```python
from build123d import *

# Parameters (mm, degrees)
F0_R     = 1
F1_DEPTH = 8
F0_W     = 23
F0_H     = 6
F2_DEPTH = 20
F4_START = -1.8
F3_W     = 10
F3_H     = 10
F3_R     = 3
F4_DEPTH = 6


with BuildPart() as f1:
    # F0 (on Top) → F1 (new body)
    with BuildSketch(Plane.XY):
        Polygon((-11.5, 1.7857142857), (-11.5, 7.7857142857), (-16.5, 7.7857142857), (-16.5, -10.2142857143), (-11.5, -10.2142857143), align=None)
        with Locations((-14, -4.7142857143)):
            Circle(F0_R, mode=Mode.SUBTRACT)
    extrude(amount=F1_DEPTH)



with BuildPart() as f1b:
    # F0 (on Top) → F1, piece 2 (new body)
    with BuildSketch(Plane.XY):
        Polygon((16.5, 7.7857142857), (11.5, 7.7857142857), (11.5, 1.7857142857), (11.5, -10.2142857143), (16.5, -10.2142857143), align=None)
        with Locations((14, -4.7142857143)):
            Circle(F0_R, mode=Mode.SUBTRACT)
    extrude(amount=F1_DEPTH)


with BuildPart() as f1_1:
    add(f1.part)

    add(f1b.part)  # F2 merges F1b
    # F0 (on Top) → F2 (join)
    with BuildSketch(Plane.XY):
        with Locations((0, 4.7857142857)):
            Rectangle(F0_W, F0_H)
    extrude(amount=F2_DEPTH)

    # F3 (on Front) → F4 (join)
    with BuildSketch(Plane.XZ.offset(F4_START)):
        with Locations((0, 25)):
            Rectangle(F3_W, F3_H)
        with Locations((0, 25)):
            Circle(F3_R, mode=Mode.SUBTRACT)
    extrude(amount=-F4_DEPTH)


solid = f1_1.part
```
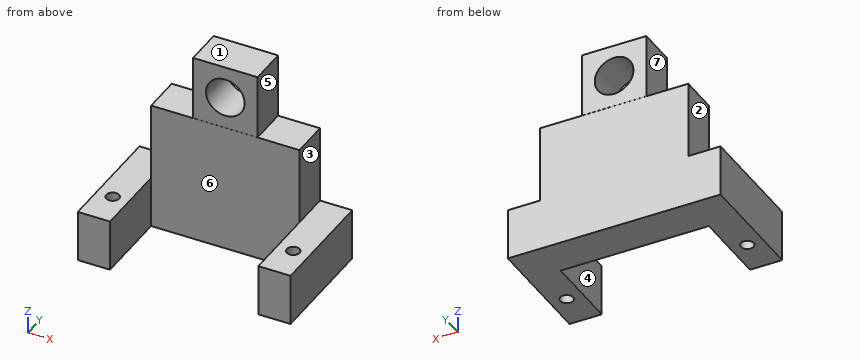
Verification items for the finished model (mm, model axes). Face numbers are marked on the shaded views. A direction names the side the tool comes from. Coordinates: 2 decimals unless noted, no trailing zeros. Loops run counter-clockwise (first coordinate to the right, second up) from the corner with the lowest first, then second, coordinate; pieces in that order, holes last. Notation, with made-up numbers: (8, 30) -> (64, 30) arc R26 ccw to (64, 50) -> close; hole circle Ø11 at (15, -8). An arc over 180 degrees is marked (long way). Answer in a Markdown table with one row per item. Add a question column.
1. Material ranges on probe 1 along Y at (x, z) = (14, 2.5); probe 2 along X at (y, z) = (-1.5, 7.5); probe 3 along Z at (x, y) = (0, 4.25), recorded low to high. Write a range as [from, to].
2. Section check A-A, the plane x = -14. Enter the section's corners in (y, z).
3. Draft check along X on the marked faces 1, 2, 3 and 4. Enter one of: +X half, -X half, draft (parallel to the pull), parting line (faces both ways), or undercut.
4. Section check D-D, the plane z = 5. Enter the section's corners in (x, y), then the cut area to 3 significant figures.
5. Section check B-B, the plane z = 25. Enter the section's corners in (x, y).
6. Access from +Z, -Z, +X, -X, +Y, -Y to the whole of each face (thin tool, end or side, straight path). Record for the marked faces 5, 6 and 7.
7. Depth check by flat-ended pin: P1, Ø10, axis at x = 2.5, z = 11.5, coming from the -Y side; P2, Ø1.8, axis at y = 6, z = 27.5, coming from the -X side; P3, Ø12, axis at x = 8.5, z = 12.5, coming from the +Y side. Enter the tip coordinate at first touch or a pass-through.
Derived:
| question | item | result |
|---|---|---|
| 1 | probe 1 | y = [-10.21, -5.71], [-3.71, 7.79] |
| 1 | probe 2 | x = [-16.5, -11.5], [11.5, 16.5] |
| 1 | probe 3 | z = [0, 22], [28, 30] |
| 2 | outline | (-10.21, 0) -> (-5.71, 0) -> (-5.71, 8) -> (-10.21, 8) -> close; (-3.71, 0) -> (7.79, 0) -> (7.79, 8) -> (-3.71, 8) -> close |
| 3 | face 1 | draft |
| 3 | face 2 | -X half |
| 3 | face 3 | +X half |
| 3 | face 4 | undercut |
| 4 | outline | (-16.5, -10.21) -> (-11.5, -10.21) -> (-11.5, 1.79) -> (11.5, 1.79) -> (11.5, -10.21) -> (16.5, -10.21) -> (16.5, 7.79) -> (-16.5, 7.79) -> close; hole circle Ø2 at (-14, -4.71); hole circle Ø2 at (14, -4.71) |
| 4 | area | 312 mm² |
| 5 | outline | (-5, 1.8) -> (-3, 1.8) -> (-3, 7.8) -> (-5, 7.8) -> close; (3, 1.8) -> (5, 1.8) -> (5, 7.8) -> (3, 7.8) -> close |
| 6 | face 5 | +Z, +X, +Y, -Y |
| 6 | face 6 | +Z, -Z, -Y |
| 6 | face 7 | +Z, -X, +Y, -Y |
| 7 | P1 | stops at y = 1.79 |
| 7 | P2 | stops at x = -5 |
| 7 | P3 | stops at y = 7.79 |
